The figure shows three views and two pictorial views of one solid part (mm, origin at its lowest corner). Answer the questions. A direction names the side the tool comes from. Round coordinates to 2 decimals unless told otherwise and drop trailing zeros. Order: outer loops, then holes, each group sorted by start corner. A loop starts at its lowest first (then second) coordinate and runs counter-clockwise, first axis right, second up.
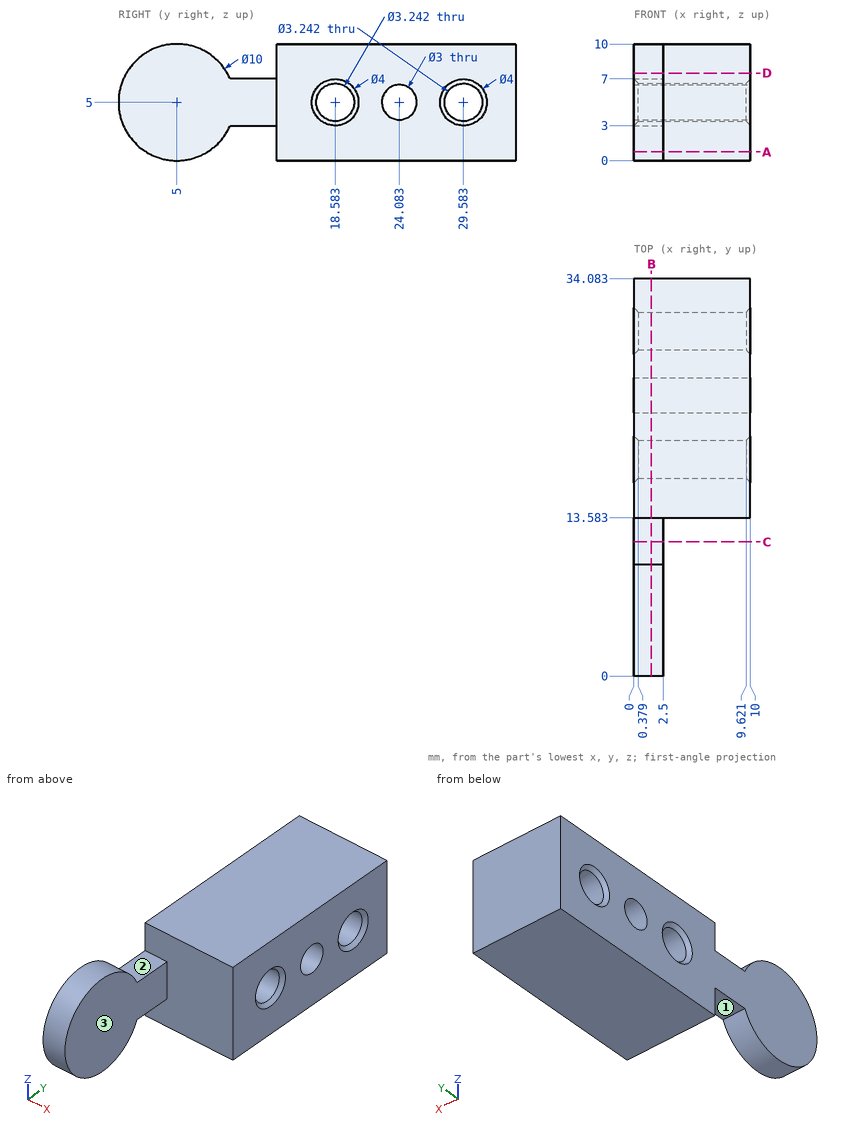
Item 1: Find section C-C (y = 11.5). Write down the section's boundary in (x, z).
Item 2: Find section B-B (x = 1.5). Write down the section's boundary in (y, z).
Item 3: Find the intervals of material crossed by line 1 along Y through (x, z) = (7, 5); line 2 along Y through (x, z) = (1.75, 4) (1 decimal); line 3 along Y through (x, z) = (1.25, 7.75) (1 decimal), in increasing order.
Item 4: Find section A-A (z = 0.75). Write down the section's boundary in (x, y).
Item 5: Given pin 1 (2.5 mm diameter, centred on y = 24.08, z = 5, fed in from +X); pin 2 (3.5 mm diameter, centred on y = 18.58, z = 5, fed in from +X); pin 3 (3 mm diameter, centred on x = 1.5, y = 11.5, fed in from +Z); pin 4 (0.8 mm diameter, centred on x = 1.5, y = 11.5, fed in from -Z), each flat-ended and moving along its own axis, determine where each tip first touches the part or whether it passes through.
Item 6: A tool of negligible diameter and unlimited length cuts with its end or side. For the marked faces 1, 2 and 3, from which of +Z, -Z, +X, -X, +Y, -Y can it reach the whole face along a straight path? Write none if from no direction.
Item 7: Find section D-D (z = 7.5). Write down the section's boundary in (x, y), plus the area to 3 significant figures.
Model answer:
1. outline: (0, 3) - (2.5, 3) - (2.5, 7) - (0, 7) - close
2. outline: (9.58, 3) - (13.58, 3) - (13.58, 0) - (34.08, 0) - (34.08, 10) - (13.58, 10) - (13.58, 7) - (9.58, 7) arc R5 ccw (long way) to start; hole circle Ø3.24 at (18.58, 5); hole circle Ø3 at (24.08, 5); hole circle Ø3.24 at (29.58, 5)
3. line 1: y = 13.58 to 16.96, 20.2 to 22.58, 25.58 to 27.96, 31.2 to 34.08
3. line 2: y = 0.1 to 17.3, 19.9 to 23, 25.2 to 28.3, 30.9 to 34.1
3. line 3: y = 0.8 to 9.2, 13.6 to 34.1
4. outline: (0, 2.37) - (2.5, 2.37) - (2.5, 7.63) - (0, 7.63) - close; (0, 13.58) - (10, 13.58) - (10, 34.08) - (0, 34.08) - close
5. pin 1: passes through
5. pin 2: stops at x = 9.75
5. pin 3: stops at z = 7
5. pin 4: stops at z = 3
6. face 1: -Z, +X, -X
6. face 2: +Z, +X, -X
6. face 3: +Z, -Z, +X, -Y
7. outline: (0, 0.67) - (2.5, 0.67) - (2.5, 9.33) - (0, 9.33) - close; (0, 13.58) - (10, 13.58) - (10, 34.08) - (0, 34.08) - close
7. area: 227 mm2
